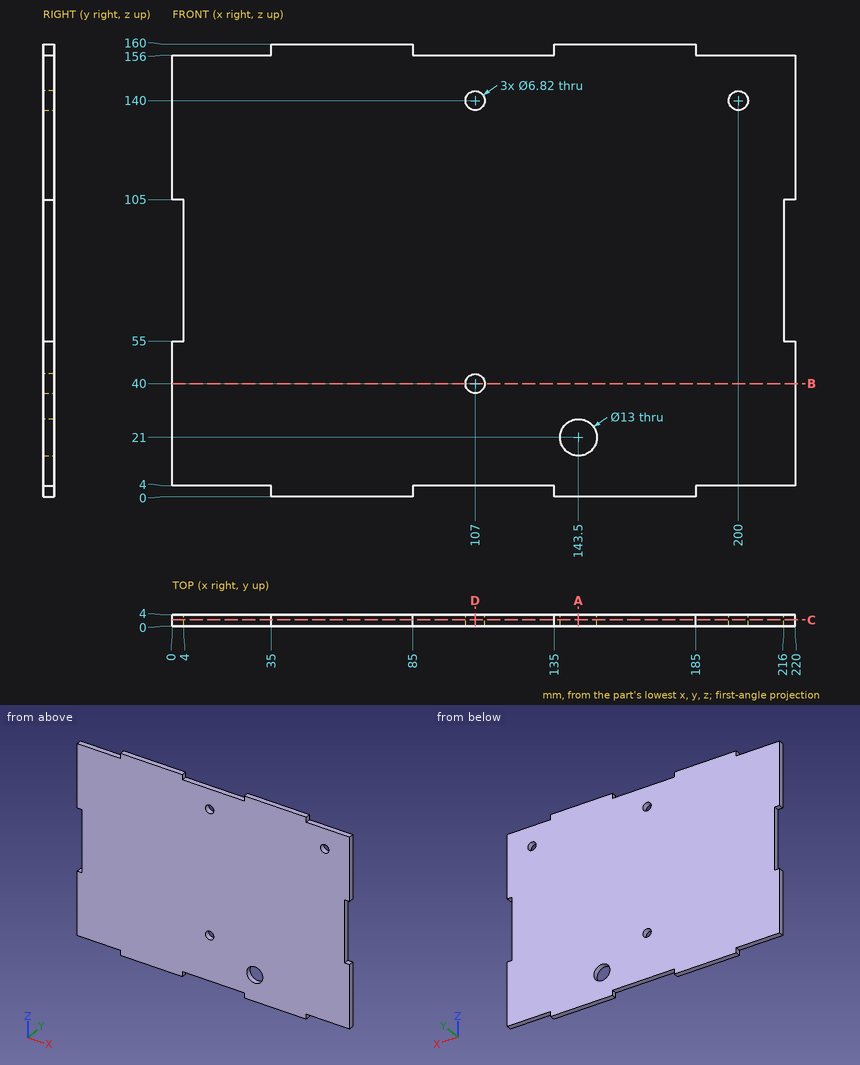
Study the drawing (mm; zero at the part's minimum x, y, z) and answer. Round coordinates to 2 decimals unless told otherwise and drop trailing zeros. Write each loop counter-clockwise with the first axis right and the second up, starting at its lowest first coordinate (ties: lowest second). Pieces come first, ordered by that corner, then holes.
Q1. Flat-ended cylindrical pins translate along their axes: P1, Ø2, axis at y = 1, z = 157.5, coming from the +X side; P2, Ø21, axis at x = 143.5, z = 21, coming from the +Y side; P3, Ø2, axis at y = 3, z = 158.5, coming from the -X side; P4, Ø2, axis at x = 121.5, y = 1, coming from the -Z side. Find the tip coordinate at first contact, or state that the pin passes through.
Values:
P1: stops at x = 185
P2: stops at y = 4
P3: stops at x = 35
P4: stops at z = 4
Q2. Find section A-A on x = 143.5. Determine the outline of the cut face in (y, z).
Values:
outline: (0, 0) - (4, 0) - (4, 14.5) - (0, 14.5) - close; (0, 27.5) - (4, 27.5) - (4, 160) - (0, 160) - close
Q3. Straight lines are drawn through the part: line 1 (X direction, y = 2.75, z = 140); line 2 (X direction, y = 2.4, z = 40); line 3 (X direction, y = 1, z = 21). For each, find the intervals that lie inside material, in ascending order.
Values:
line 1: x = 0 to 103.59, 110.41 to 196.59, 203.41 to 220
line 2: x = 0 to 103.59, 110.41 to 220
line 3: x = 0 to 137, 150 to 220
Q4. Find section D-D on x = 107. Determine the outline of the cut face in (y, z), and give its area (3 significant figures).
Values:
outline: (0, 4) - (4, 4) - (4, 36.59) - (0, 36.59) - close; (0, 43.41) - (4, 43.41) - (4, 136.59) - (0, 136.59) - close; (0, 143.41) - (4, 143.41) - (4, 156) - (0, 156) - close
area: 553 mm2
Q5. Find section C-C on y = 2.25. State how many separate pieces and enclosed holes the cut face has, and give its area (3 significant figures).
Values:
separate pieces: 1
enclosed holes: 4
area: 33,600 mm2
Q6. Find section B-B on z = 40. Determine the outline of the cut face in (x, y), and give its area (3 significant figures).
Values:
outline: (0, 0) - (103.59, 0) - (103.59, 4) - (0, 4) - close; (110.41, 0) - (220, 0) - (220, 4) - (110.41, 4) - close
area: 853 mm2
